The model under review builds one solid part; all positions refer to its coordinate system, in mm. A direction names the side the tool comes from. Round coordinates to 2 decimals unless told otherwise and drop trailing zeros. Order: outer loops, then holes, each group sorted by start corner. A loop starts at its lowest first (then second) coordinate and runs counter-clockwise, first axis right, second up.
1) Clearance check with flat-ended pins moving along their axes: P1, Ø4.5, axis at x = 13, y = -5, coming from the +Z side; P2, Ø4.5, axis at x = -20, z = 24, coming from the -Y side; P3, Ø3, axis at x = -12.5, y = -10.5, coming from the -Z side. State where each tip first meets the part, or that it passes through.
2) Consider section D-D (z = -12). Give the boundary of the cut face in (x, y), then the cut area to 3 significant figures.
3) Consider section B-B (y = -5). Give the boundary of the cut face in (x, z), then the cut area to 3 significant figures.
4) Machinability: for faces 1 (the face through (-11, 12.5, 0)), 2 (the face through (-31, -20, 0)), 3 (the face through (-41, -7, -7.5)), 4 (the face through (10, -4, 0)), which of the approach directions +Z, -Z, +X, -X, +Y, -Y give a long, thin tool a straight path to every point of the face, cutting with its end or side? Answer none if there is none.
5) Consider section A-A (x = -30). Give the boundary of the cut face in (y, z).
6) Consider section C-C (z = -29). Give the boundary of the cut face in (x, y), then the cut area to 4 significant figures.
7) Mouldability with a two-part tool opening along X and no side actions: class faces 5 (the face through (-1, 6, 35)), 6 (the face through (-16.134, -22.465, 21.041)), 7 (the face through (-31.69, 6.16, 25.84)) as pulls with the +X half, pulls with the -X half, needs draft (parallel to the pull), parting line crosses it, or undercut.
8) To check wall thickness, follow L1, parallel to X at y = 7.5, z = -7; L2, parallel to X at y = 8, z = -24; L3, parallel to Y at x = -30, z = 31.5. State the ranges of each line that lie inside material, in increasing order.
from build123d import *

# Parameters (mm, degrees)
SKETCH1_W           = 90
SKETCH1_H           = 70
SKETCH1_R           = 2.5
SKETCH1_W_2         = 22
SKETCH1_H_2         = 42
BOSS_EXTRUDE1_DEPTH = 12.5
SKETCH3_W           = 9
SKETCH3_H           = 15
SKETCH3_W_2         = 28
BOSS_EXTRUDE2_DEPTH = 15
SKETCH4_W           = 20
SKETCH4_H           = 20
CUT_EXTRUDE1_DEPTH  = 64.294944506
SKETCH7_W           = 90
SKETCH7_H           = 70
SKETCH7_W_2         = 20
SKETCH7_H_2         = 20
BOSS_EXTRUDE3_DEPTH = 5
SKETCH8_R           = 26.514354508
SKETCH8_R_2         = 2.5
BOSS_EXTRUDE4_DEPTH = 5


with BuildPart() as part:
    # Sketch1 → Boss-Extrude1 (new body)
    with BuildSketch(Plane(origin=(0, 0, 0), x_dir=(1, 0, 0), z_dir=(0, 1, 0))):
        Rectangle(SKETCH1_W, SKETCH1_H)
        with Locations(Location((-30, 24, 0), (0, 0, 270))):
            Circle(SKETCH1_R, mode=Mode.SUBTRACT)
        with Locations(Location((-20, 24, 0), (0, 0, 270))):
            Circle(SKETCH1_R, mode=Mode.SUBTRACT)
        with Locations(Location((-20, -24, 0), (0, 0, 90))):
            Circle(SKETCH1_R, mode=Mode.SUBTRACT)
        with Locations(Location((-30, -24, 0), (0, 0, 90))):
            Circle(SKETCH1_R, mode=Mode.SUBTRACT)
        with Locations(Location((20, -24, 0), (0, 0, 270))):
            Circle(SKETCH1_R, mode=Mode.SUBTRACT)
        with Locations(Location((30, -24, 0), (0, 0, 270))):
            Circle(SKETCH1_R, mode=Mode.SUBTRACT)
        with Locations(Location((20, 24, 0), (0, 0, 90))):
            Circle(SKETCH1_R, mode=Mode.SUBTRACT)
        with Locations(Location((30, 24, 0), (0, 0, 90))):
            Circle(SKETCH1_R, mode=Mode.SUBTRACT)
        with Locations((-25, 0)):
            Rectangle(SKETCH1_W_2, SKETCH1_H_2, mode=Mode.SUBTRACT)
        with Locations((25, 0)):
            Rectangle(SKETCH1_W_2, SKETCH1_H_2, mode=Mode.SUBTRACT)
    extrude(amount=BOSS_EXTRUDE1_DEPTH)

    # Sketch3 → Boss-Extrude2 (add)
    with BuildSketch(Plane.XZ):
        with Locations((-40.5, 0)):
            Rectangle(SKETCH3_W, SKETCH3_H)
        Rectangle(SKETCH3_W_2, SKETCH3_H)
        with Locations((40.5, 0)):
            Rectangle(SKETCH3_W, SKETCH3_H)
    extrude(amount=BOSS_EXTRUDE2_DEPTH)

    # Sketch4 → Cut-Extrude1 (cut, through all)
    with BuildSketch(Plane(origin=(0, 12.5, 0), x_dir=(1, 0, 0), z_dir=(0, 1, 0))):
        Rectangle(SKETCH4_W, SKETCH4_H)
    extrude(amount=-CUT_EXTRUDE1_DEPTH, mode=Mode.SUBTRACT)

    # Sketch7 → Boss-Extrude3 (add)
    with BuildSketch(Plane.XZ.offset(15)):
        Rectangle(SKETCH7_W, SKETCH7_H)
        Rectangle(SKETCH7_W_2, SKETCH7_H_2, mode=Mode.SUBTRACT)
    extrude(amount=BOSS_EXTRUDE3_DEPTH)

    # Sketch8 → Boss-Extrude4 (add)
    with BuildSketch(Plane.XZ.offset(20)):
        with Locations(Location((0, 0, 0), (0, 0, 270))):
            Circle(SKETCH8_R)
        with Locations(Location((0, 0, 0), (0, 0, 270))):
            Circle(SKETCH8_R_2, mode=Mode.SUBTRACT)
    extrude(amount=BOSS_EXTRUDE4_DEPTH)


solid = part.part
Answer below:
1. P1: stops at z = 7.5
1. P2: stops at y = -20
1. P3: stops at z = -7.5
2. outline: (-45, -20) - (-23.64, -20) - (-23.64, -25) - (23.64, -25) - (23.64, -20) - (45, -20) - (45, -15) - (-45, -15) - close; (-45, 0) - (-36, 0) - (-36, 12.5) - (-45, 12.5) - close; (-14, 0) - (14, 0) - (14, 12.5) - (-14, 12.5) - close; (36, 0) - (45, 0) - (45, 12.5) - (36, 12.5) - close
2. area: 1,260 mm2
3. outline: (-45, -7.5) - (-36, -7.5) - (-36, 7.5) - (-45, 7.5) - close; (-14, -7.5) - (-10, -7.5) - (-10, 7.5) - (-14, 7.5) - close; (10, -7.5) - (14, -7.5) - (14, 7.5) - (10, 7.5) - close; (36, -7.5) - (45, -7.5) - (45, 7.5) - (36, 7.5) - close
3. area: 390 mm2
4. face 1: +Z, -Z, +X, -X, +Y
4. face 2: -Y
4. face 3: -Z, +X, -X
4. face 4: +Y
5. outline: (-20, -35) - (-15, -35) - (-15, 35) - (-20, 35) - close; (0, -35) - (12.5, -35) - (12.5, -26.5) - (0, -26.5) - close; (0, -21.5) - (12.5, -21.5) - (12.5, -21) - (0, -21) - close; (0, 21) - (12.5, 21) - (12.5, 21.5) - (0, 21.5) - close; (0, 26.5) - (12.5, 26.5) - (12.5, 35) - (0, 35) - close
6. outline: (-45, -20) - (45, -20) - (45, -15) - (-45, -15) - close; (-45, 0) - (45, 0) - (45, 12.5) - (-45, 12.5) - close
6. area: 1,575 mm2
7. face 5: needs draft
7. face 6: parting line crosses it
7. face 7: undercut
8. L1: x = -45 to -36, -14 to -10, 10 to 14, 36 to 45
8. L2: x = -45 to -32.5, -27.5 to -22.5, -17.5 to 17.5, 22.5 to 27.5, 32.5 to 45
8. L3: y = -20 to -15, 0 to 12.5
